```python
from build123d import *

# Parameters (mm, degrees)
F0_R     = 18.5
F1_DEPTH = 2.5
F2_R     = 15.5
F3_DEPTH = 10
F4_R     = 13.25
F5_DEPTH = 5
F6_R     = 10
F7_DEPTH = 7.501


with BuildPart() as f1:
    # F0 (on Top) → F1 (new body)
    with BuildSketch(Plane.XY):
        Circle(F0_R)
    extrude(amount=F1_DEPTH)

    # F2 (on face) → F3 (join)
    with BuildSketch(Plane.XY.offset(2.5)):
        Circle(F2_R)
    extrude(amount=F3_DEPTH)

    # F4 (on face) → F5 (cut)
    with BuildSketch(Plane(origin=(0, 0, 0), x_dir=(1, 0, 0), z_dir=(0, 0, -1))):
        Circle(F4_R)
    extrude(amount=-F5_DEPTH, mode=Mode.SUBTRACT)

    # F6 (on face) → F7 (cut, through all)
    with BuildSketch(Plane(origin=(0, 0, 5), x_dir=(1, 0, 0), z_dir=(0, 0, -1))):
        Circle(F6_R)
    extrude(amount=-F7_DEPTH, mode=Mode.SUBTRACT)


solid = f1.part
```
Geometry: final body of the model. Coordinates: model frame, mm. A direction names the side the tool comes from. Give positions to 0.01 mm unless a question says otherwise; leave off trailing zeros. Loops run counter-clockwise (first coordinate to the right, second up) from the corner with the lowest first, then second, coordinate; pieces in that order, holes last. Notation, with made-up numbers: (11.25, 55.25) -> (45.25, 55.25) arc R31 ccw to (45.25, 91.25) -> close; hole circle Ø2 at (-36, 87). An arc over 180 degrees is marked (long way). Use one line per item in the form item = value.
Item 1: Line query: probe 1 along Y at (x, z) = (0, 2.05); probe 2 along Y at (x, z) = (0, 7.5); probe 3 along X at (y, z) = (-0.5, 4.25). Output: solid intervals per line, ascending.
A:
probe_1 = -18.5 to -13.25, 13.25 to 18.5
probe_2 = -15.5 to -10, 10 to 15.5
probe_3 = -15.49 to -13.24, 13.24 to 15.49
Item 2: Draft query along X for faces 1 (the face through (-2.17, 9.76, 8.7)), 2 (the face through (-4.01, -18.06, 1.23)), 3 (the face through (8, -14, 2.5)). Return one class per face: pulls with the +X half, pulls with the -X half, needs draft (parallel to the pull), parting line crosses it, or undercut.
A:
face_1 = undercut
face_2 = parting line crosses it
face_3 = needs draft
Item 3: Section query A-A on y = 0. Output: boundary loops of the cut face in (x, z).
A:
outline = (-18.5, 0) -> (-13.25, 0) -> (-13.25, 5) -> (-10, 5) -> (-10, 12.5) -> (-15.5, 12.5) -> (-15.5, 2.5) -> (-18.5, 2.5) -> close; (10, 5) -> (13.25, 5) -> (13.25, 0) -> (18.5, 0) -> (18.5, 2.5) -> (15.5, 2.5) -> (15.5, 12.5) -> (10, 12.5) -> close
Item 4: Section query C-C on z = 4.25. Output: boundary loops of the cut face in (x, y), and give its area (3 significant figures).
A:
outline = circle Ø31 at (0, 0); hole circle Ø26.5 at (0, 0)
area = 203 mm^2
Item 5: Pin query (flat end, axial travel): P1, Ø1, axis at x = 6, z = 4.5, coming from the +Y side; P2, Ø2, axis at x = 4, z = 4.5, coming from the -Y side; P3, Ø1.5, axis at x = 7.5, z = 7, coming from the -Y side; P4, Ø16, axis at x = 0, y = 0, coming from the +Z side. Return the tip coordinate at first contact, or that it passes through.
A:
P1 = 14.49
P2 = -15.21
P3 = -13.95
P4 = through
Item 6: Section query D-D on x = 12.5. Output: boundary loops of the cut face in (y, z).
A:
outline = (-13.64, 0) -> (-4.39, 0) -> (-4.39, 5) -> (4.39, 5) -> (4.39, 0) -> (13.64, 0) -> (13.64, 2.5) -> (9.17, 2.5) -> (9.17, 12.5) -> (-9.17, 12.5) -> (-9.17, 2.5) -> (-13.64, 2.5) -> close
Item 7: Access query for faces 4 (the face through (-2.018, 15.368, 7.43)), 5 (the face through (7.123, -11.172, 2.465)), 6 (the face through (-4, 13, 0)). Directions: +Z, -Z, +X, -X, +Y, -Y. A direction counts if a zero-diameter tool reaches every point of the face in a straight line with its end or side. Return the directions, or none.
A:
face_4 = +Z
face_5 = -Z
face_6 = -Z, +X, -X, +Y, -Y
